Part model, mm, in its own coordinate system. A direction names the side the tool comes from. Coordinates: 2 decimals unless noted, no trailing zeros. Loops run counter-clockwise (first coordinate to the right, second up) from the corner with the lowest first, then second, coordinate; pieces in that order, holes last. Notation, with made-up numbers: M 5.5,1 L 23.5,1 A13 ccw 23.5,18 Z; hole C 60.5,73.25 d5. An arc over 180 degrees is marked long. Answer as a JSON object with one key per item and string values. Group by question number.
1. Saw through at B-B on y = 255. Write the cut outline in (x, z), then the cut area to 3 significant figures.
2. Saw through at D-D on y = -301.5. Write the cut outline in (x, z).
3. Saw through at C-C on x = 116.5. Write the cut outline in (y, z).
4. Drop flat-ended pins along their axis: pin 1 Ø5 at (x, y) = (-100.5, -68) entering from +Z; pin 2 Ø12 at (x, z) = (3, 52) entering from +Y; pin 3 Ø4 at (x, z) = (-142.5, 1006) entering from +Y. Give the stop position or say it passes through.
5. 3-axis set-ups, long thin cutter, end or side, ignore diameter. For faces 1 (the face through (-4, -485, 619)), 2 (the face through (10.41, 509.65, 1009.32)), 3 (the face through (-3.47, 239.38, 1267.32)): which of +Z, -Z, +X, -X, +Y, -Y reach the whole face in a straight line?
6. Drill centre lines: L1, parallel to Z at x = -150.5, y = 115; L2, parallel to Y at x = 238, z = 795.5. Where is each one in solid material? Low to high.
7. Saw through at A-A on z = 930. Write the cut outline in (x, y), then the cut area to 3 significant figures.
from build123d import *

# Parameters (mm, degrees)
F0_W     = 520
F0_H     = 970
F1_DEPTH = 1255
F2_R     = 80
F3_DEPTH = 50
F5_R     = 7.5
F6_DEPTH = 20
F7_R     = 16
F8_DEPTH = 25


# Not quite as in the source:
# - the program builds the solid bodies; features that only make, move or delete a surface that nothing else refers to are left out


with BuildPart() as f1:
    # F0 (on Top) → F1 (new body)
    with BuildSketch(Plane.XY):
        Rectangle(F0_W, F0_H)
    extrude(amount=F1_DEPTH)

    # F2 (on face) → F3 (join)
    with BuildSketch(Plane(origin=(0, 485, 0), x_dir=(-1, 0, 0), z_dir=(0, 1, 0))):
        with Locations((0, 930)):
            Circle(F2_R)
    extrude(amount=F3_DEPTH)

    # F5 (on face) → F6 (join)
    with BuildSketch(Plane(origin=(0, 485, 0), x_dir=(-1, 0, 0), z_dir=(0, 1, 0))):
        with Locations((0, 52.045196724)):
            Circle(F5_R)
    extrude(amount=F6_DEPTH)

    # F7 (on face) → F8 (join)
    with BuildSketch(Plane.XY.offset(1255)):
        with Locations((0, 255)):
            Circle(F7_R)
    extrude(amount=F8_DEPTH)


solid = f1.part
Outcome:
{
 "1": {"outline": "M -260,0 L 260,0 L 260,1255 L 16,1255 L 16,1280 L -16,1280 L -16,1255 L -260,1255 Z", "area": "653,000 mm²"},
 "2": {"outline": "M -260,0 L 260,0 L 260,1255 L -260,1255 Z"},
 "3": {"outline": "M -485,0 L 485,0 L 485,1255 L -485,1255 Z"},
 "4": {"pin 1": "stops at z = 1255", "pin 2": "stops at y = 505", "pin 3": "stops at y = 485"},
 "5": {"face 1": "+Z, -Z, +X, -X, -Y", "face 2": "+Y", "face 3": "+Z"},
 "6": {"L1": "z = 0 to 1255", "L2": "y = -485 to 485"},
 "7": {"outline": "M -260,-485 L 260,-485 L 260,485 L 80,485 L 80,535 L -80,535 L -80,485 L -260,485 Z", "area": "512,000 mm²"}
}
